Work out the finished part from the listing and answer in its coordinate system (mm). A direction names the side the tool comes from. Give positions to 0.01 mm unless a question says otherwise; leave off trailing zeros. Order: outer loops, then holes, each group sorted by start corner. A loop starts at its lowest first (then second) coordinate and runs counter-clockwise, first axis right, second up. Notation, with made-up numbers: (-23, 77.5) - (-16, 77.5) arc R26 cw to (-16, 109.5) - close; hole circle Ø1 at (2.5, 13.25). An arc over 180 degrees is marked (long way). Write each question's results on one line, items separated by ' | '.
from build123d import *

# Parameters (mm, degrees)
IZIM1_W                     = 72
IZIM1_H                     = 56
Y_KSEKLIK_EKSTR_ZYON2_DEPTH = 1
IZIM3_W                     = 72
IZIM3_H                     = 56
IZIM3_W_2                   = 70
IZIM3_H_2                   = 54
EKSTR_ZYON_NCE2_DEPTH       = 13
IZIM4_W                     = 10
IZIM4_H                     = 4
KES_EKSTR_ZYON1_DEPTH       = 1
IZIM5_R                     = 2
KES_EKSTR_ZYON2_DEPTH       = 1
IZIM6_W                     = 1
IZIM6_H                     = 14
Y_KSEKLIK_EKSTR_ZYON3_DEPTH = 56
IZIM7_W                     = 10
IZIM7_H                     = 3
KES_EKSTR_ZYON3_DEPTH       = 1
IZIM8_W                     = 74
IZIM8_H                     = 58
IZIM8_W_2                   = 72
IZIM8_H_2                   = 56
EKSTR_ZYON_NCE4_DEPTH       = 13
IZIM9_W                     = 10
IZIM9_H                     = 5
KES_EKSTR_ZYON4_DEPTH       = 1
IZIM10_W                    = 10
IZIM10_H                    = 1.5
Y_KSEKLIK_EKSTR_ZYON4_DEPTH = 2
IZIM11_W                    = 10
IZIM11_H                    = 3.5
KES_EKSTR_ZYON5_DEPTH       = 2
IZIM12_W                    = 74
IZIM12_H                    = 58
IZIM12_W_2                  = 72
IZIM12_H_2                  = 56
EKSTR_ZYON_NCE5_DEPTH       = 1


with BuildPart() as part:
    # Çizim1 → Yükseklik-Ekstrüzyon2 (new body)
    with BuildSketch(Plane(origin=(0, 0, 0), x_dir=(1, 0, 0), z_dir=(0, 1, 0))):
        Rectangle(IZIM1_W, IZIM1_H)
    extrude(amount=Y_KSEKLIK_EKSTR_ZYON2_DEPTH)

    # Çizim3 → Ekstrüzyon-İnce2 (add)
    with BuildSketch(Plane(origin=(0, 1, 0), x_dir=(1, 0, 0), z_dir=(0, 1, 0))):
        Rectangle(IZIM3_W, IZIM3_H)
        Rectangle(IZIM3_W_2, IZIM3_H_2, mode=Mode.SUBTRACT)
    extrude(amount=EKSTR_ZYON_NCE2_DEPTH)

    # Çizim4 → Kes-Ekstrüzyon1 (cut)
    with BuildSketch(Plane.ZY.offset(-35)):
        with Locations((20.9, 4)):
            Rectangle(IZIM4_W, IZIM4_H)
    extrude(amount=-KES_EKSTR_ZYON1_DEPTH, mode=Mode.SUBTRACT)

    # Çizim5 → Kes-Ekstrüzyon2 (cut)
    with BuildSketch(Plane(origin=(0, 1, 0), x_dir=(1, 0, 0), z_dir=(0, 1, 0))):
        with Locations(Location((19.5, -24, 0), (0, 0, 270))):
            Circle(IZIM5_R)
        with Locations(Location((22, 24.5, 0), (0, 0, 270))):
            Circle(IZIM5_R)
        with Locations(Location((-31, -9, 0), (0, 0, 270))):
            Circle(IZIM5_R)
        with Locations(Location((-31, 20, 0), (0, 0, 270))):
            Circle(IZIM5_R)
    extrude(amount=-KES_EKSTR_ZYON2_DEPTH, mode=Mode.SUBTRACT)

    # Çizim6 → Yükseklik-Ekstrüzyon3 (add)
    with BuildSketch(Plane.XY.offset(28)):
        with Locations((35.5, 7)):
            Rectangle(IZIM6_W, IZIM6_H)
    extrude(amount=-Y_KSEKLIK_EKSTR_ZYON3_DEPTH)

    # Çizim7 → Kes-Ekstrüzyon3 (cut)
    with BuildSketch(Plane.ZY.offset(-35)):
        with Locations((11, 3.7)):
            Rectangle(IZIM7_W, IZIM7_H)
    extrude(amount=-KES_EKSTR_ZYON3_DEPTH, mode=Mode.SUBTRACT)

    # Çizim8 → Ekstrüzyon-İnce4 (add)
    with BuildSketch(Plane(origin=(0, 1, 0), x_dir=(1, 0, 0), z_dir=(0, 1, 0))):
        Rectangle(IZIM8_W, IZIM8_H)
        Rectangle(IZIM8_W_2, IZIM8_H_2, mode=Mode.SUBTRACT)
    extrude(amount=EKSTR_ZYON_NCE4_DEPTH)

    # Çizim9 → Kes-Ekstrüzyon4 (cut)
    with BuildSketch(Plane.ZY.offset(-35)):
        with Locations((11, 4.7)):
            Rectangle(IZIM9_W, IZIM9_H)
    extrude(amount=-KES_EKSTR_ZYON4_DEPTH, mode=Mode.SUBTRACT)

    # Çizim10 → Yükseklik-Ekstrüzyon4 (add)
    with BuildSketch(Plane.ZY.offset(-35)):
        with Locations((11, 2.95)):
            Rectangle(IZIM10_W, IZIM10_H)
    extrude(amount=-Y_KSEKLIK_EKSTR_ZYON4_DEPTH)

    # Çizim11 → Kes-Ekstrüzyon5 (cut)
    with BuildSketch(Plane.ZY.offset(-35)):
        with Locations((11, 5.45)):
            Rectangle(IZIM11_W, IZIM11_H)
    extrude(amount=-KES_EKSTR_ZYON5_DEPTH, mode=Mode.SUBTRACT)

    # Çizim12 → Ekstrüzyon-İnce5 (add)
    with BuildSketch(Plane.XZ.offset(-1)):
        Rectangle(IZIM12_W, IZIM12_H)
        Rectangle(IZIM12_W_2, IZIM12_H_2, mode=Mode.SUBTRACT)
    extrude(amount=EKSTR_ZYON_NCE5_DEPTH)


solid = part.part
1. Straight lines are drawn through the part: line 1 (X direction, y = 0.65, z = 9); line 2 (X direction, y = 13, z = -18.5); line 3 (Z direction, x = 2, y = 6.25). For each, find the intervals that lie inside material, in ascending order. Write a range as [from, to].
Answer list:
line 1: [-37, -33], [-29, 37] | line 2: [-37, -35], [35, 37] | line 3: [-29, -27], [27, 29]
2. Determine the mould class of faces 1 (the face through (-1, 7, -29)), 2 (the face through (36, 5, 16)), 3 (the face through (-3, 14, 28)), 4 (the face through (-1, 0, 0)) for opening direction Y: +Y half, -Y half, draft (parallel to the pull), parting line (faces both ways), or undercut.
Answer list:
face 1: draft | face 2: undercut | face 3: +Y half | face 4: -Y half
3. A cutting plane is placed at C-C, the plane y = 12.5. Write down the section's boundary in (x, z).
Answer list:
outline: (-37, -29) - (37, -29) - (37, 29) - (-37, 29) - close; hole (-35, -27) - (35, -27) - (35, 27) - (-35, 27) - close
4. A cutting plane is placed at A-A, the plane z = 12. Write down the section's boundary in (x, y), then the cut area to 3 significant figures.
Answer list:
outline: (-37, 0) - (37, 0) - (37, 3.7) - (35, 3.7) - (35, 1) - (-35, 1) - (-35, 14) - (-37, 14) - close; (35, 7.2) - (37, 7.2) - (37, 14) - (35, 14) - close | area: 119 mm^2
5. A cutting plane is placed at B-B, the plane x = -31. Write down the section's boundary in (y, z), then the cut area to 3 significant figures.
Answer list:
outline: (0, -29) - (14, -29) - (14, -27) - (1, -27) - (1, -22) - (0, -22) - close; (0, -18) - (1, -18) - (1, 7) - (0, 7) - close; (0, 11) - (1, 11) - (1, 27) - (14, 27) - (14, 29) - (0, 29) - close | area: 102 mm^2
6. A cutting plane is placed at D-D, the plane z = 5. Write down the section's boundary in (x, y).
Answer list:
outline: (-37, 0) - (37, 0) - (37, 14) - (35, 14) - (35, 1) - (-35, 1) - (-35, 14) - (-37, 14) - close
7. A tool of negligible diameter and unlimited length cuts with its end or side. For faces 5 (the face through (0, 7, 27)), 6 (the face through (36, 3.7, 11)), 7 (the face through (-37, 7, 0)), from which of +Z, -Z, +X, -X, +Y, -Y can it reach the whole face along a straight path? Write none if from no direction.
Answer list:
face 5: +Y | face 6: +X | face 7: +Z, -Z, -X, +Y, -Y
8. Given P1, Ø3, axis at x = -5.5, z = 16, coming from the +Y side, flat-ended and moving along its own axis, determine where the tip first touches the part or whether it passes through.
Answer list:
P1: y = 1
